For this review, take the finished solid that the model builds, in its own axes (mm). Face numbers are marked on the shaded views. A direction names the side the tool comes from. Give positions to 0.01 mm unless a question says otherwise; leave off trailing zeros. Order: outer loops, then holes, each group sorted by start corner. A loop starts at its lowest first (then second) coordinate and runs counter-clockwise, first axis right, second up. Notation, with made-up numbers: (28, 23.5) - (64, 23.5) arc R25 cw to (64, 40.5) - close; hole circle Ø2 at (36.5, 45.25). An arc over 180 degrees is marked (long way). One line per item, written item: value.
```python
from build123d import *

# Parameters (mm, degrees)
SKETCH_1_R      = 37.5
SKETCH_1_R_2    = 3
EXTRUDE_1_DEPTH = 5
EXTRUDE_START   = 10
SKETCH_2_R      = 37.5
EXTRUDE_2_DEPTH = 10
SKETCH_3_R      = 37.5
SKETCH_3_R_2    = 1
SKETCH_3_W      = 12
SKETCH_3_H      = 12
EXTRUDE_3_DEPTH = 5
SKETCH_4_R      = 37.5
SKETCH_4_R_2    = 1
SKETCH_4_W      = 12
SKETCH_4_H      = 25
EXTRUDE_4_DEPTH = 2
SKETCH_5_R      = 37.5
SKETCH_5_R_2    = 20
SKETCH_5_R_3    = 1
EXTRUDE_5_DEPTH = 2


with BuildPart() as part:
    # Эскиз1 → Бобышка-Вытянуть1 (new body)
    with BuildSketch(Plane.XY):
        Circle(SKETCH_1_R)
        Circle(SKETCH_1_R_2, mode=Mode.SUBTRACT)
    extrude(amount=EXTRUDE_1_DEPTH)

    # Эскиз2 → Бобышка-Вытянуть2 (add)
    with BuildSketch(Plane(origin=(0, 0, 0), x_dir=(-1, 0, 0), z_dir=(0, 0, -1)).offset(EXTRUDE_START)):
        Circle(SKETCH_2_R)
    extrude(amount=-EXTRUDE_2_DEPTH)

    # Эскиз3 → Бобышка-Вытянуть3 (add)
    with BuildSketch(Plane.XY.offset(5)):
        with Locations(Location((0, 0, 0), (0, 0, 180))):
            Circle(SKETCH_3_R)
        with Locations((0, 30)):
            Circle(SKETCH_3_R_2, mode=Mode.SUBTRACT)
        with Locations((0, -30)):
            Circle(SKETCH_3_R_2, mode=Mode.SUBTRACT)
        with Locations((-30, 0)):
            Circle(SKETCH_3_R_2, mode=Mode.SUBTRACT)
        with Locations((30, 0)):
            Circle(SKETCH_3_R_2, mode=Mode.SUBTRACT)
        with Locations((-23, 21)):
            Circle(SKETCH_3_R_2, mode=Mode.SUBTRACT)
        with Locations((-23, -21)):
            Circle(SKETCH_3_R_2, mode=Mode.SUBTRACT)
        with Locations((23, -21)):
            Circle(SKETCH_3_R_2, mode=Mode.SUBTRACT)
        with Locations((23, 21)):
            Circle(SKETCH_3_R_2, mode=Mode.SUBTRACT)
        Rectangle(SKETCH_3_W, SKETCH_3_H, mode=Mode.SUBTRACT)
    extrude(amount=EXTRUDE_3_DEPTH)

    # Эскиз4 → Бобышка-Вытянуть4 (add)
    with BuildSketch(Plane.XY.offset(10)):
        with Locations(Location((0, 0, 0), (0, 0, 180))):
            Circle(SKETCH_4_R)
        with Locations((0, 30)):
            Circle(SKETCH_4_R_2, mode=Mode.SUBTRACT)
        with Locations((0, -30)):
            Circle(SKETCH_4_R_2, mode=Mode.SUBTRACT)
        with Locations((-30, 0)):
            Circle(SKETCH_4_R_2, mode=Mode.SUBTRACT)
        with Locations((30, 0)):
            Circle(SKETCH_4_R_2, mode=Mode.SUBTRACT)
        with Locations((-23, -21)):
            Circle(SKETCH_4_R_2, mode=Mode.SUBTRACT)
        with Locations((23, -21)):
            Circle(SKETCH_4_R_2, mode=Mode.SUBTRACT)
        with Locations((-23, 21)):
            Circle(SKETCH_4_R_2, mode=Mode.SUBTRACT)
        with Locations((23, 21)):
            Circle(SKETCH_4_R_2, mode=Mode.SUBTRACT)
        Rectangle(SKETCH_4_W, SKETCH_4_H, mode=Mode.SUBTRACT)
    extrude(amount=EXTRUDE_4_DEPTH)

    # Эскиз5 → Бобышка-Вытянуть5 (add)
    with BuildSketch(Plane.XY.offset(12)):
        with Locations(Location((0, 0, 0), (0, 0, 180))):
            Circle(SKETCH_5_R)
        Circle(SKETCH_5_R_2, mode=Mode.SUBTRACT)
        with Locations((0, 30)):
            Circle(SKETCH_5_R_3, mode=Mode.SUBTRACT)
        with Locations((0, -30)):
            Circle(SKETCH_5_R_3, mode=Mode.SUBTRACT)
        with Locations((-30, 0)):
            Circle(SKETCH_5_R_3, mode=Mode.SUBTRACT)
        with Locations((30, 0)):
            Circle(SKETCH_5_R_3, mode=Mode.SUBTRACT)
        with Locations((-23, 21)):
            Circle(SKETCH_5_R_3, mode=Mode.SUBTRACT)
        with Locations((23, 21)):
            Circle(SKETCH_5_R_3, mode=Mode.SUBTRACT)
        with Locations((-23, -21)):
            Circle(SKETCH_5_R_3, mode=Mode.SUBTRACT)
        with Locations((23, -21)):
            Circle(SKETCH_5_R_3, mode=Mode.SUBTRACT)
    extrude(amount=EXTRUDE_5_DEPTH)


solid = part.part
```
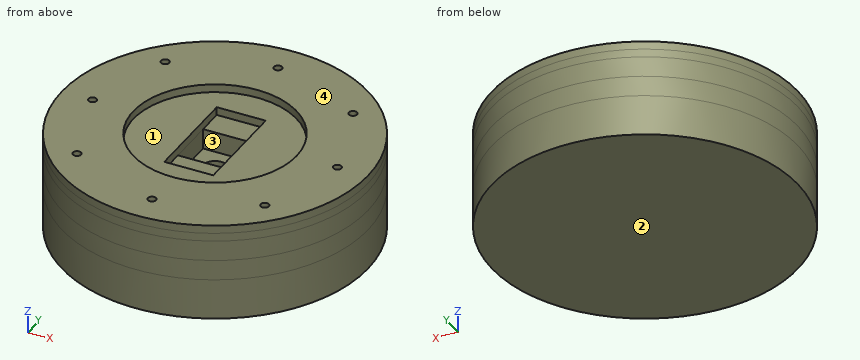
(1) Draft analysis for pull direction X (two halves, no side actions). For the marked faces 1 and 2, state which applies: pulls with the +X half, pulls with the -X half, needs draft (parallel to the pull), parting line crosses it, or undercut.
Answers below:
face 1: undercut
face 2: needs draft
(2) Take a section at B-B (z = 9). Give the number of separate pieces and of enclosed holes in the cut face, then the cut area to 3 significant figures.
Answers below:
separate pieces: 1
enclosed holes: 9
area: 4,250 mm^2
(3) Take a section at C-C (y = -30). Write out the cut boundary in (x, z).
Answers below:
outline: (-22.5, -10) - (22.5, -10) - (22.5, 14) - (1, 14) - (1, 5) - (-1, 5) - (-1, 14) - (-22.5, 14) - close
(4) Take a section at A-A (x = 0). Write out the cut boundary in (y, z), then the cut area to 3 significant figures.
Answers below:
outline: (-37.5, -10) - (37.5, -10) - (37.5, 14) - (31, 14) - (31, 5) - (29, 5) - (29, 14) - (20, 14) - (20, 12) - (12.5, 12) - (12.5, 10) - (6, 10) - (6, 5) - (3, 5) - (3, 0) - (-3, 0) - (-3, 5) - (-6, 5) - (-6, 10) - (-12.5, 10) - (-12.5, 12) - (-20, 12) - (-20, 14) - (-29, 14) - (-29, 5) - (-31, 5) - (-31, 14) - (-37.5, 14) - close
area: 1,540 mm^2
(5) Machinability: for the marked faces 3 and 4, which of the approach directions +Z, -Z, +X, -X, +Y, -Y give a long, thin tool a straight path to every point of the face, cutting with its end or side? Answer none if there is none.
Answers below:
face 3: +Z
face 4: +Z, +X, -X, +Y, -Y
(6) Wall thickness on line 1 (Y direction, x = 0, z = 11.4); line 2 (Y direction, x = 0, z = 7.35); line 3 (Y direction, x = -30, z = 13.45): over which ranges is each line inside the solid? List them lowest first. Write a range as from..to.
Answers below:
line 1: y = -37.5..-31, -29..-12.5, 12.5..29, 31..37.5
line 2: y = -37.5..-31, -29..-6, 6..29, 31..37.5
line 3: y = -22.5..-1, 1..22.5
(7) Take a section at D-D (z = 1). Write out the cut boundary in (x, y).
Answers below:
outline: circle Ø75 at (0, 0); hole circle Ø6 at (0, 0)
(8) For P1, Ø1.6, axis at x = 23, y = -21, coming from the +Z side; P2, Ø2, axis at x = 1, y = 9.5, coming from the +Z side; P3, Ø12, axis at x = 3.5, z = 10, coming from the +Y side; P4, Ø2.5, axis at x = -23, y = 21, coming from the +Z side, all flat-tipped, find the tip position at first contact; note any pin that passes through.
Answers below:
P1: stops at z = 5
P2: stops at z = 10
P3: stops at y = 37.5
P4: stops at z = 14
